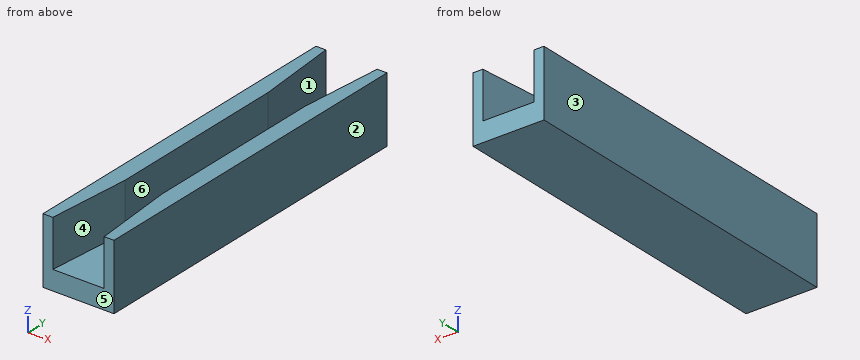
```python
from build123d import *

# Parameters (mm, degrees)
F1_DEPTH   = 105
F2_SIZE2   = 4.3744331763
F2_SIZE    = 50
F2_2_SIZE2 = 4.3744331763
F2_2_SIZE  = 50
F3_SIZE2   = 4.3744331763
F3_SIZE    = 50


with BuildPart() as f1:
    # F0 (on Front) → F1 (new body, symmetric)
    with BuildSketch(Plane.XZ):
        Polygon((-11, 28), (-21.25, 28), (-21.25, -11.6291716302), (21.25, -11.6291716302), (21.25, 27.8708283698), (11, 27.8708283698), (11, 0), (-11, 0), align=None)
    extrude(amount=F1_DEPTH, both=True)

    # F2
    f2_edges = [f1.edges().sort_by_distance(p)[0] for p in [
        (-11, -105, 14),
        (-11, 105, 14),
    ]]
    f2_side = f1.faces().sort_by_distance((-11, 0, 14))[0]
    chamfer(f2_edges, length=F2_SIZE, length2=F2_SIZE2, reference=f2_side)

    # F2#2
    f2_2_edges = [f1.edges().sort_by_distance(p)[0] for p in [
        (11, -105, 13.935414),
    ]]
    f2_2_side = f1.faces().sort_by_distance((11, 0, 13.935414))[0]
    chamfer(f2_2_edges, length=F2_2_SIZE, length2=F2_2_SIZE2, reference=f2_2_side)

    # F3
    f3_edges = [f1.edges().sort_by_distance(p)[0] for p in [
        (11, 105, 13.935414),
    ]]
    f3_side = f1.faces().sort_by_distance((11, 25, 13.935414))[0]
    chamfer(f3_edges, length=F3_SIZE, length2=F3_SIZE2, reference=f3_side)


solid = f1.part
```
Verification items for the finished model (mm, model axes). Face numbers are marked on the shaded views. A direction names the side the tool comes from. Round coordinates to 2 decimals unless told otherwise and drop trailing zeros. Order: outer loops, then holes, each group sorted by start corner. A loop starts at its lowest first (then second) coordinate and runs counter-clockwise, first axis right, second up.
1) Draft check along X on the marked faces 3, 4, 5 and 6. Enter one of: +X half, -X half, draft (parallel to the pull), parting line (faces both ways), or undercut.
Geometry says:
face 3: -X half
face 4: undercut
face 5: draft
face 6: undercut
2) Cross-section at C-C, the plane x = -13.5. Record the cut outline in (y, z).
Geometry says:
outline: (-105, -11.63) - (105, -11.63) - (105, 0) - (83.58, 0) - (83.58, 28) - (-83.58, 28) - (-83.58, 0) - (-105, 0) - close
3) Cross-section at B-B, the plane y = 2.5. Record the cut outline in (x, z), plus the area to 3 significant figures.
Geometry says:
outline: (-21.25, -11.63) - (21.25, -11.63) - (21.25, 27.87) - (11, 27.87) - (11, 0) - (-11, 0) - (-11, 28) - (-21.25, 28) - close
area: 1,070 mm2
4) Cross-section at A-A, the plane z = 19.5. Record the cut outline in (x, y).
Geometry says:
outline: (-21.25, -105) - (-15.37, -105) - (-11, -55) - (-11, 55) - (-15.37, 105) - (-21.25, 105) - close; (11, -55) - (15.37, -105) - (21.25, -105) - (21.25, 105) - (15.37, 105) - (11, 55) - close
5) Tool access check on the marked faces 1 and 2. Record the directions out of +Z, -Z, +X, -X, +Y, -Y that give a thin tool (end or side, any length) a straight path to the whole face; none if there is none.
Geometry says:
face 1: +Z, +Y
face 2: +Z, -Z, +X, +Y, -Y
6) Depth check by flat-ended pin: pin 1 (15.5 mm diameter, centred on x = -5.5, y = 35, fed in from +Z); pin 2 (8 mm diameter, centred on x = 14.5, y = 0, fed in from +Z). Enter the tip coordinate at first touch or a pass-through.
Geometry says:
pin 1: stops at z = 28
pin 2: stops at z = 27.87
7) Cross-section at D-D, the plane x = 4. Record the cut outline in (y, z), plus the area to 3 significant figures.
Geometry says:
outline: (-105, -11.63) - (105, -11.63) - (105, 0) - (-105, 0) - close
area: 2,440 mm2
8) Material ranges on line 1 (X direction, y = 3, z = 5.5); line 2 (Z direction, x = 0, y = -50); line 3 (X direction, y = 57.5, z = 14.5), recorded low to high.
Geometry says:
line 1: x = -21.25 to -11, 11 to 21.25
line 2: z = -11.63 to 0
line 3: x = -21.25 to -11.22, 11.22 to 21.25
